For this review, take the finished solid that the model builds, in its own axes (mm). A direction names the side the tool comes from. Round coordinates to 2 decimals unless told otherwise and drop trailing zeros. Order: outer loops, then holes, each group sorted by start corner. A loop starts at its lowest first (then second) coordinate and runs counter-clockwise, first axis right, second up. Notation, with made-up numbers: M 31,-10.75 L 84,-10.75 A10 ccw 84,3.25 Z; hole C -3,89.25 d8. An arc over 180 degrees is marked long. Answer in a Markdown table with one row per item. Add a question column.
```python
from build123d import *

# Parameters (mm, degrees)
SKETCH1_R           = 60
BOSS_EXTRUDE1_DEPTH = 10
SKETCH2_R           = 5
BOSS_EXTRUDE2_DEPTH = 40
SKETCH5_R           = 5
CUT_EXTRUDE1_DEPTH  = 10
SKETCH6_W           = 10
SKETCH6_H           = 5
BOSS_EXTRUDE4_DEPTH = 10


with BuildPart() as part:
    # Sketch1 → Boss-Extrude1 (new body)
    with BuildSketch(Plane.XY):
        Circle(SKETCH1_R)
    extrude(amount=BOSS_EXTRUDE1_DEPTH)

    # Sketch2 → Boss-Extrude2 (add)
    with BuildSketch(Plane.XY.offset(10)):
        Circle(SKETCH2_R)
    extrude(amount=BOSS_EXTRUDE2_DEPTH)

    # Sketch5 → Cut-Extrude1 (cut)
    with BuildSketch(Plane(origin=(0, 0, 0), x_dir=(-1, 0, 0), z_dir=(0, 0, -1))):
        with Locations((0, -30)):
            Circle(SKETCH5_R)
    extrude(amount=-CUT_EXTRUDE1_DEPTH, mode=Mode.SUBTRACT)

    # Sketch6 → Boss-Extrude4 (add)
    with BuildSketch(Plane(origin=(0, 0, 0), x_dir=(-1, 0, 0), z_dir=(0, 0, -1))):
        with Locations((40, 32.5)):
            Rectangle(SKETCH6_W, SKETCH6_H)
        with Locations((-40, 32.5)):
            Rectangle(SKETCH6_W, SKETCH6_H)
    extrude(amount=BOSS_EXTRUDE4_DEPTH)


solid = part.part
```
1. Consider section A-A on x = 0. Write out the cut boundary in (y, z), plus the area to 3 significant figures.
2. For faces 1 (the flat face through (-35, 32, -5)), 2 (the flat face through (40, 35, -5)), 3 (the flat face through (45, 32, -5)), 4 (the cylindrical face through (-1.08, -4.88, 29.72)), list the 3-axis set-ups (+Z, -Z, +X, -X, +Y, -Y) from which the entire face can be reached by the end or side of a thin tool; tool diameter is ignored.
3. The part is to be moulded in two halves that separate along X. For faces 5 (the flat face through (40, 30, -5)), 6 (the flat face through (-45, 32, -5)), 7 (the flat face through (35, 32, -5)), say which applies: pulls with the +X half, pulls with the -X half, needs draft (parallel to the pull), parting line crosses it, or undercut.
4. Consider section C-C on y = -30. Write out the cut boundary in (x, z), plus the area to 3 significant figures.
5. To check wall thickness, follow probe 1 along Y at (x, z) = (0, 6); probe 2 along Z at (x, y) = (29.5, 0); probe 3 along X at (y, z) = (-37, 7). State the ranges of each line that lie inside material, in increasing order. Write a range as [from, to].
6. Consider section B-B on z = -3.5. Write out the cut boundary in (x, y), plus the area to 3 significant figures.
7. Consider section D-D on z = 3. Write out the cut boundary in (x, y).
8. Clearance check with flat-ended pins moving along their axes: pin 1 Ø1.5 at (x, y) = (30.5, 24.5) entering from -Z; pin 2 Ø11 at (x, z) = (40.5, -6.5) entering from +Y; pin 3 Ø1.5 at (y, z) = (32, -6) entering from -X. State where each tip first meets the part, or that it passes through.
Solved:
| question | item | result |
|---|---|---|
| 1 | outline | M -60,0 L -35,0 L -35,10 L -60,10 Z; M -25,0 L 60,0 L 60,10 L 5,10 L 5,50 L -5,50 L -5,10 L -25,10 Z |
| 1 | area | 1,500 mm^2 |
| 2 | face 1 | -Z, +Y, -Y |
| 2 | face 2 | -Z, +X, -X, +Y |
| 2 | face 3 | -Z, +X, +Y, -Y |
| 2 | face 4 | +Z |
| 3 | face 5 | needs draft |
| 3 | face 6 | pulls with the -X half |
| 3 | face 7 | undercut |
| 4 | outline | M -51.96,0 L -5,0 L -5,10 L -51.96,10 Z; M 5,0 L 51.96,0 L 51.96,10 L 5,10 Z |
| 4 | area | 939 mm^2 |
| 5 | probe 1 | y = [-60, -35], [-25, 60] |
| 5 | probe 2 | z = [0, 10] |
| 5 | probe 3 | x = [-47.23, 47.23] |
| 6 | outline | M -45,30 L -35,30 L -35,35 L -45,35 Z; M 35,30 L 45,30 L 45,35 L 35,35 Z |
| 6 | area | 100 mm^2 |
| 7 | outline | C 0,0 d120; hole C 0,-30 d10 |
| 8 | pin 1 | stops at z = 0 |
| 8 | pin 2 | stops at y = 35 |
| 8 | pin 3 | stops at x = -45 |
